Build history of the part. All positions in model axes, mm. Face numbers are marked on the shaded views. A direction names the side the tool comes from. Round coordinates to 2 decimals unless told otherwise and drop trailing zeros. Order: outer loops, then holes, each group sorted by start corner. A loop starts at its lowest first (then second) coordinate and runs counter-clockwise, first axis right, second up. Notation, with made-up numbers: M 65,74 L 114,74 A20 cw 114,87 Z; hole C -22.75,-11.75 d5. An arc over 180 degrees is marked long. Use CSV: the item, a comma, the result in double quotes.
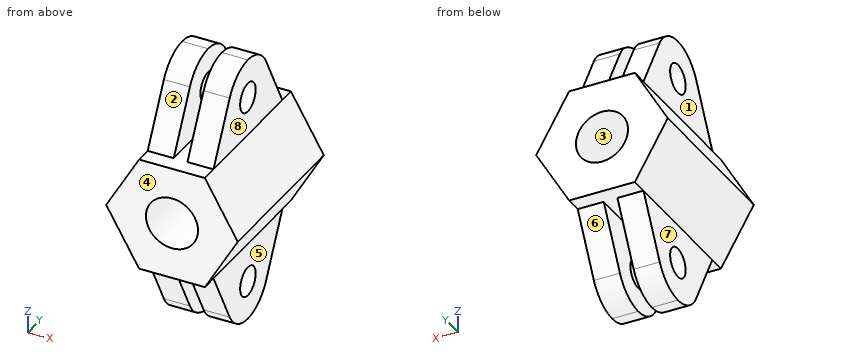
from build123d import *

# Parameters (mm, degrees)
F0_R      = 8
F1_DEPTH  = 25
F2_W      = 20.2072594216
F2_H      = 40
F3_DEPTH  = 24
F4_R      = 4.5
F5_DEPTH  = 30.3118891325
F7_DEPTH  = 25.4
F8_W      = 4.2072594216
F8_H      = 50
F9_DEPTH  = 25.4
F10_W     = 20.2072594216
F10_H     = 40
F11_DEPTH = 24
F12_R     = 4.5
F13_DEPTH = 25.4
F15_DEPTH = 25.4
F16_W     = 4.2072594216
F16_H     = 50
F17_DEPTH = 25.4


with BuildPart() as f1:
    # F0 (on Front) → F1 (new body, symmetric)
    with BuildSketch(Plane.XZ):
        Polygon((10.1036297108, 17.5), (-10.1036297108, 17.5), (-20.2072594216, 0), (-10.1036297108, -17.5), (10.1036297108, -17.5), (20.2072594216, 0), align=None)
        Circle(F0_R, mode=Mode.SUBTRACT)
    extrude(amount=F1_DEPTH, both=True)

    # F2 (on face) → F3 (join)
    with BuildSketch(Plane.XY.offset(17.5)):
        Rectangle(F2_W, F2_H)
    extrude(amount=F3_DEPTH)

    # F4 (on face) → F5 (cut, through all)
    with BuildSketch(Plane(origin=(-10.1036297108, 0, 0), x_dir=(0, -1, 0), z_dir=(-1, 0, 0))):
        with Locations((0, 29.5)):
            Circle(F4_R)
    extrude(amount=-F5_DEPTH, mode=Mode.SUBTRACT)

    # F6 (on face) → F7 (cut)
    with BuildSketch(Plane(origin=(-10.1036297108, 0, 0), x_dir=(0, -1, 0), z_dir=(-1, 0, 0))):
        with BuildLine():
            Line((-20, 41.5), (-20, 17.5))
            Line((-20, 17.5), (-10.5882352941, 35.1470588235))
            ThreePointArc((-10.5882352941, 35.1470588235), (-6.1739490436, 39.7899151215), (5.03e-08, 41.5))
            Line((5.03e-08, 41.5), (-20, 41.5))
        make_face()
        with BuildLine():
            Line((10.5882352941, 35.1470588235), (20, 17.5))
            Line((20, 17.5), (20, 41.5))
            Line((20, 41.5), (5.03e-08, 41.5))
            ThreePointArc((5.03e-08, 41.5), (6.1739490867, 39.7899150956), (10.5882352941, 35.1470588235))
        make_face()
    extrude(amount=-F7_DEPTH, mode=Mode.SUBTRACT)

    # F8 (on face) → F9 (cut)
    with BuildSketch(Plane.XY.offset(17.5)):
        Rectangle(F8_W, F8_H)
    extrude(amount=F9_DEPTH, mode=Mode.SUBTRACT)

    # F10 (on face) → F11 (join)
    with BuildSketch(Plane(origin=(0, 0, -17.5), x_dir=(1, 0, 0), z_dir=(0, 0, -1))):
        Rectangle(F10_W, F10_H)
    extrude(amount=F11_DEPTH)

    # F12 (on face) → F13 (cut)
    with BuildSketch(Plane.YZ.offset(10.1036297108)):
        with Locations((0, -29.5)):
            Circle(F12_R)
    extrude(amount=-F13_DEPTH, mode=Mode.SUBTRACT)

    # F14 (on face) → F15 (cut)
    with BuildSketch(Plane.YZ.offset(10.1036297108)):
        with BuildLine():
            Line((20, -41.5), (20, -17.5))
            Line((20, -17.5), (10.5882352941, -35.1470588235))
            ThreePointArc((10.5882352941, -35.1470588235), (6.1739490436, -39.7899151215), (-5.03e-08, -41.5))
            Line((-5.03e-08, -41.5), (20, -41.5))
        make_face()
        with BuildLine():
            Line((-10.5882352941, -35.1470588235), (-20, -17.5))
            Line((-20, -17.5), (-20, -41.5))
            Line((-20, -41.5), (-5.03e-08, -41.5))
            ThreePointArc((-5.03e-08, -41.5), (-6.1739490867, -39.7899150956), (-10.5882352941, -35.1470588235))
        make_face()
    extrude(amount=-F15_DEPTH, mode=Mode.SUBTRACT)

    # F16 (on face) → F17 (cut)
    with BuildSketch(Plane(origin=(0, 0, -17.5), x_dir=(1, 0, 0), z_dir=(0, 0, -1))):
        Rectangle(F16_W, F16_H)
    extrude(amount=F17_DEPTH, mode=Mode.SUBTRACT)


solid = f1.part
(1) Drop flat-ended pins along their axis: pin 1 (1.5 mm diameter, centred on x = -1.5, z = 29.5, fed in from -Y); pin 2 (10.5 mm diameter, centred on y = 0, z = -29.5, fed in from +X); pin 3 (4 mm diameter, centred on x = 10, y = -5, fed in from +Z); pin 4 (16 mm diameter, centred on x = 4, y = -3.5, fed in from +Z). Give the stop position or say it passes through.
Answer block:
pin 1,"stops at y = -13.84"
pin 2,"stops at x = 10.1"
pin 3,"stops at z = 41.12"
pin 4,"stops at z = 41.5"
(2) Cut at C-C, the plane z = -4.5. Give the cut face in (x, y).
Answer block:
outline,"M -17.61,-25 L -6.61,-25 L -6.61,25 L -17.61,25 Z; M 6.61,-25 L 17.61,-25 L 17.61,25 L 6.61,25 Z"
(3) Tool access for the marked faces 4, 5, 6, 7 and 8: list every direction of +Z, -Z, +X, -X, +Y, -Y with a clear straight run to the whole face (end or side of a thin tool).
Answer block:
face 4,"+Z, -Z, +X, -X, -Y"
face 5,"-Z, +X, +Y, -Y"
face 6,"-Z, +X, -X, +Y"
face 7,"-Z, -X, +Y, -Y"
face 8,"+Z, +X, +Y, -Y"
(4) Two-plate mould, pull along X, no slides. Class the marked faces 1, 2 and 3: released by +X, released by -X, zero draft, split by the parting line, or undercut.
Answer block:
face 1,"released by -X"
face 2,"zero draft"
face 3,"undercut"
(5) Cut at A-A, the plane z = -29.5. Give the cut face in (x, y), and give its area (3 significant figures).
Answer block:
outline,"M -10.1,-13.6 L -2.1,-13.6 L -2.1,-4.5 L -10.1,-4.5 Z; M -10.1,4.5 L -2.1,4.5 L -2.1,13.6 L -10.1,13.6 Z; M 2.1,-13.6 L 10.1,-13.6 L 10.1,-4.5 L 2.1,-4.5 Z; M 2.1,4.5 L 10.1,4.5 L 10.1,13.6 L 2.1,13.6 Z"
area,"291 mm²"
(6) Wall check: line 1 (X direction, y = 12, z = 31.5); line 2 (Z direction, x = -6.5, y = 0); line 3 (Z direction, x = 6, y = 0). Give the ranges that are in metal, low to high. Write a range as from..to.
Answer block:
line 1,"x = -10.1..-2.1, 2.1..10.1"
line 2,"z = -41.5..-34, -25..-4.66, 4.66..25, 34..41.5"
line 3,"z = -41.5..-34, -25..-5.29, 5.29..25, 34..41.5"
(7) Cut at D-D, the plane y = -9. Give the cut face in (x, z).
Answer block:
outline,"M -20.21,0 L -10.1,-17.5 L -10.1,-37.44 L -2.1,-37.44 L -2.1,-17.5 L 2.1,-17.5 L 2.1,-37.44 L 10.1,-37.44 L 10.1,-17.5 L 20.21,0 L 10.1,17.5 L 10.1,37.44 L 2.1,37.44 L 2.1,17.5 L -2.1,17.5 L -2.1,37.44 L -10.1,37.44 L -10.1,17.5 Z; hole C 0,0 d16"
(8) Cut at B-B, the plane x = 0. Give the cut face in (y, z), and give its area (3 significant figures).
Answer block:
outline,"M -25,-17.5 L 25,-17.5 L 25,-8 L -25,-8 Z; M -25,8 L 25,8 L 25,17.5 L -25,17.5 Z"
area,"950 mm²"
